Geometry check sheet. Reference: the model listing, model coordinates, mm. Face numbers are marked on the shaded views. Round coordinates to 2 decimals unless told otherwise and drop trailing zeros. Write each loop counter-clockwise with the first axis right and the second up, starting at its lowest first coordinate (ties: lowest second). Pieces come first, ordered by that corner, then holes. Notation, with made-up numbers: M 83,83.25 L 97,83.25 A38 ccw 97,122.25 Z; hole C 70,-30 d1. An arc over 180 degrees is marked long. One line per item, written item: value. Start each with the question number.
1. Release check for a two-part mould opening along Y. For the marked faces 1, 2 and 3 record: pulls with the +Y half, pulls with the -Y half, needs draft (parallel to the pull), parting line crosses it, or undercut.
2. Depth check by flat-ended pin: P1, Ø1, axis at y = 28.5, z = -2, coming from the -X side; P2, Ø4, axis at x = 1, y = 7.5, coming from the -Z side; P3, Ø3, axis at x = 3, y = 41.5, coming from the +Z side. Enter the tip coordinate at first touch or a pass-through.
3. Section check C-C (y = 0.5). Record the boundary of the cut face in (x, z).
4. Scan lines: probe 1 along Y at (x, z) = (0.75, 2.5); probe 2 along Y at (x, z) = (0, 3); probe 3 along X at (y, z) = (3.5, 0). Record each from-to range of solid material in increasing order. Write a range as [from, to].
5. Section check B-B (z = -1.5). Record the boundary of the cut face in (x, y).
6. Section check A-A (x = 0). Record the boundary of the cut face in (y, z).
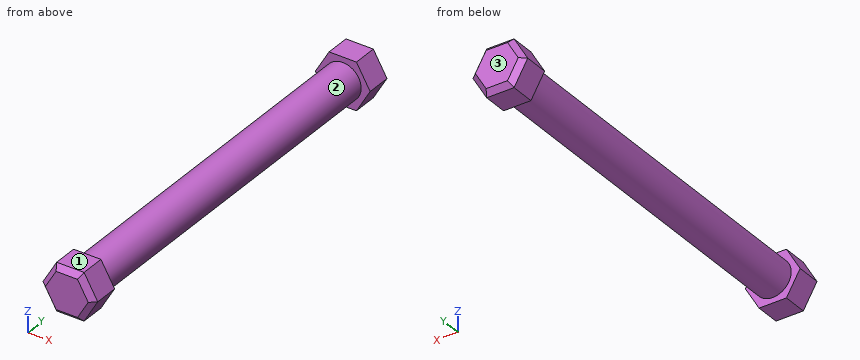
from build123d import *

# Parameters (mm, degrees)
SKETCH1_R           = 2.5
BOSS_EXTRUDE1_DEPTH = 50
BOSS_EXTRUDE2_DEPTH = 4
CHAMFER1_SIZE       = 0.7
BOSS_EXTRUDE3_DEPTH = 4
CHAMFER2_SIZE       = 0.7


with BuildPart() as part:
    # Sketch1 → Boss-Extrude1 (new body)
    with BuildSketch(Plane(origin=(0, 0, 0), x_dir=(1, 0, 0), z_dir=(0, 1, 0))):
        Circle(SKETCH1_R)
    extrude(amount=BOSS_EXTRUDE1_DEPTH)

    # Sketch2 → Boss-Extrude2 (add)
    with BuildSketch(Plane(origin=(0, 50, 0), x_dir=(1, 0, 0), z_dir=(0, 1, 0))):
        Polygon((3.720037117, 0), (1.860018559, 3.221646647), (-1.860018559, 3.221646647), (-3.720037117, 0), (-1.860018559, -3.221646647), (1.860018559, -3.221646647), align=None)
    extrude(amount=BOSS_EXTRUDE2_DEPTH)

    # Chamfer1
    chamfer1_edges = [part.edges().sort_by_distance(p)[0] for p in [
        (2.790027838, 54, 1.610823323),
        (2.790027838, 54, -1.610823323),
        (0, 54, -3.221646647),
        (-2.790027838, 54, -1.610823323),
        (-2.790027838, 54, 1.610823323),
        (0, 54, 3.221646647),
    ]]
    chamfer(chamfer1_edges, length=CHAMFER1_SIZE)

    # Sketch3 → Boss-Extrude3 (add)
    with BuildSketch(Plane.XZ):
        Polygon((3.720037117, 0), (1.860018559, 3.221646647), (-1.860018559, 3.221646647), (-3.720037117, 0), (-1.860018559, -3.221646647), (1.860018559, -3.221646647), align=None)
    extrude(amount=BOSS_EXTRUDE3_DEPTH)

    # Chamfer2
    chamfer2_edges = [part.edges().sort_by_distance(p)[0] for p in [
        (2.790027838, -4, -1.610823323),
        (2.790027838, -4, 1.610823323),
        (0, -4, 3.221646647),
        (-2.790027838, -4, 1.610823323),
        (-2.790027838, -4, -1.610823323),
        (0, -4, -3.221646647),
    ]]
    chamfer(chamfer2_edges, length=CHAMFER2_SIZE)


solid = part.part
Result sheet:
1. face 1: needs draft
1. face 2: undercut
1. face 3: pulls with the +Y half
2. P1: stops at x = -2
2. P2: stops at z = -2.5
2. P3: stops at z = 2
3. outline: C 0,0 d5
4. probe 1: y = [-4, 0], [50, 54]
4. probe 2: y = [-3.52, 0], [50, 53.52]
4. probe 3: x = [-2.5, 2.5]
5. outline: M -2.85,-3.3 L -2.05,-4 L 2.05,-4 L 2.85,-3.3 L 2.85,0 L 2,0 L 2,50 L 2.85,50 L 2.85,53.3 L 2.05,54 L -2.05,54 L -2.85,53.3 L -2.85,50 L -2,50 L -2,0 L -2.85,0 Z
6. outline: M -4,-2.52 L -3.3,-3.22 L 0,-3.22 L 0,-2.5 L 50,-2.5 L 50,-3.22 L 53.3,-3.22 L 54,-2.52 L 54,2.52 L 53.3,3.22 L 50,3.22 L 50,2.5 L 0,2.5 L 0,3.22 L -3.3,3.22 L -4,2.52 Z
